```python
from build123d import *

# Parameters (mm, degrees)
PAD_DEPTH       = 36
SKETCH001_R     = 4.2
POCKET_DEPTH    = 28.001
SKETCH002_R     = 16.5
POCKET001_DEPTH = 10
POCKET002_DEPTH = 6.5
SKETCH004_R     = 11.25
POCKET003_DEPTH = 1.5
SKETCH005_R     = 2.7
POCKET004_DEPTH = 10
SKETCH006_R     = 4.75
POCKET005_DEPTH = 1
CHAMFER_SIZE    = 3
CHAMFER001_SIZE = 4
CHAMFER002_SIZE = 6
CHAMFER003_SIZE = 3
CHAMFER004_SIZE = 0.8
CHAMFER005_SIZE = 1
CHAMFER006_SIZE = 0.6
CHAMFER007_SIZE = 0.4


with BuildPart() as part:
    # Sketch (on XZ_Plane of Origin) → Pad (new body, symmetric)
    with BuildSketch(Plane.XZ):
        Polygon((0, 0), (0, 20), (-37, 20), (-37, -8), (20, -8), (20, 0), align=None)
    extrude(amount=PAD_DEPTH, both=True)

    # Sketch001 (on Face2 of Pad) → Pocket (cut, through all)
    with BuildSketch(Plane.XY.offset(20)):
        with Locations((-18.5, 0)):
            Circle(SKETCH001_R)
    extrude(amount=-POCKET_DEPTH, mode=Mode.SUBTRACT)

    # Sketch002 (on Face9 of Pocket) → Pocket001 (cut)
    with BuildSketch(Plane(origin=(0, 0, -8), x_dir=(1, 0, 0), z_dir=(0, 0, -1))):
        with Locations((-18.5, 0)):
            Circle(SKETCH002_R)
    extrude(amount=-POCKET001_DEPTH, mode=Mode.SUBTRACT)

    # Sketch003 (on Face10 of Pocket001) → Pocket002 (cut)
    with BuildSketch(Plane(origin=(0, 0, 2), x_dir=(1, 0, 0), z_dir=(0, 0, -1))):
        Polygon((-10.994447, 0), (-14.747223, 6.5), (-22.252777, 6.5), (-26.005553, 0), (-22.252777, -6.5), (-14.747223, -6.5), align=None)
    extrude(amount=-POCKET002_DEPTH, mode=Mode.SUBTRACT)

    # Sketch004 (on Face3 of Pocket002) → Pocket003 (cut)
    with BuildSketch(Plane.XY.offset(20)):
        with Locations((-18.5, 0)):
            Circle(SKETCH004_R)
    extrude(amount=-POCKET003_DEPTH, mode=Mode.SUBTRACT)

    # Sketch005 (on Face2 of Pocket003) → Pocket004 (cut)
    with BuildSketch(Plane.XY):
        with Locations((10, -26)):
            Circle(SKETCH005_R)
        with Locations((10, 26)):
            Circle(SKETCH005_R)
    extrude(amount=-POCKET004_DEPTH, mode=Mode.SUBTRACT)

    # Sketch006 (on Face11 of Pocket004) → Pocket005 (cut)
    with BuildSketch(Plane(origin=(0, 0, -8), x_dir=(1, 0, 0), z_dir=(0, 0, -1))):
        with Locations((10, 26)):
            Circle(SKETCH006_R)
        with Locations((10, -26)):
            Circle(SKETCH006_R)
    extrude(amount=-POCKET005_DEPTH, mode=Mode.SUBTRACT)

    # Chamfer
    chamfer_edges = [part.edges().sort_by_distance(p)[0] for p in [
        (0, -36, 10),
        (0, 36, 10),
    ]]
    chamfer(chamfer_edges, length=CHAMFER_SIZE)

    # Chamfer001
    chamfer001_edges = [part.edges().sort_by_distance(p)[0] for p in [
        (20, -36, -4),
        (20, 36, -4),
    ]]
    chamfer(chamfer001_edges, length=CHAMFER001_SIZE)

    # Chamfer002
    chamfer002_edges = [part.edges().sort_by_distance(p)[0] for p in [
        (-37, -36, 6),
        (-37, 36, 6),
    ]]
    chamfer(chamfer002_edges, length=CHAMFER002_SIZE)

    # Chamfer003
    chamfer003_edges = [part.edges().sort_by_distance(p)[0] for p in [
        (-35, 0, 2),
    ]]
    chamfer(chamfer003_edges, length=CHAMFER003_SIZE)

    # Chamfer004
    chamfer004_edges = [part.edges().sort_by_distance(p)[0] for p in [
        (-35, 0, -8),
    ]]
    chamfer(chamfer004_edges, length=CHAMFER004_SIZE)

    # Chamfer005
    chamfer005_edges = [part.edges().sort_by_distance(p)[0] for p in [
        (-22.7, 0, 18.5),
        (-22.7, 0, 8.5),
    ]]
    chamfer(chamfer005_edges, length=CHAMFER005_SIZE)

    # Chamfer006
    chamfer006_edges = [part.edges().sort_by_distance(p)[0] for p in [
        (7.3, 26, -7),
        (7.3, -26, -7),
        (7.3, -26, 0),
        (7.3, 26, 0),
    ]]
    chamfer(chamfer006_edges, length=CHAMFER006_SIZE)

    # Chamfer007
    chamfer007_edges = [part.edges().sort_by_distance(p)[0] for p in [
        (-17, 36, 20),
        (-34, 33, 20),
        (-1.5, 34.5, 20),
        (-37, 0, 20),
        (0, 0, 20),
        (-34, -33, 20),
        (-1.5, -34.5, 20),
        (-17, -36, 20),
        (-29.75, 0, 20),
        (-35.8, 0, -8),
        (-7.5, 36, -8),
        (-34, 33, -8),
        (18, 34, -8),
        (-37, 0, -8),
        (20, 0, -8),
        (-34, -33, -8),
        (18, -34, -8),
        (-7.5, -36, -8),
        (5.25, -26, -8),
        (5.25, 26, -8),
    ]]
    chamfer(chamfer007_edges, length=CHAMFER007_SIZE)


solid = part.part
```
Part model, mm, in its own coordinate system. A direction names the side the tool comes from. Round coordinates to 2 decimals unless told otherwise and drop trailing zeros. Order: outer loops, then holes, each group sorted by start corner. A loop starts at its lowest first (then second) coordinate and runs counter-clockwise, first axis right, second up. Notation, with made-up numbers: M 20.5,35 L 39.5,35 A30 ccw 39.5,58 Z; hole C 28.5,36 d4. An arc over 180 degrees is marked long. Put each result on its own line as item: value. Start each with the question number.
1. Slice it at C-C on z = 14. List the corners of the cut face in (x, y).
2. Slice it at B-B on x = 10. State how many separate pieces and enclosed holes the cut face has, then the cut area to 3 significant figures.
3. Drill centre lines: probe 1 along Y at (x, z) = (10, -3.6); probe 2 along Y at (x, z) = (10, -7.2); probe 3 along Y at (x, z) = (-18.5, 18.7). Where is each one in solid material? Low to high. Write a range as [from, to].
4. Drop flat-ended pins along their axis: pin 1 (7 mm diameter, centred on x = 8.5, y = -1, fed in from +Z); pin 2 (6.5 mm diameter, centred on x = -18.5, y = 0, fed in from +Z); pin 3 (6.5 mm diameter, centred on x = -17, y = -3, fed in from -Z); pin 4 (7 mm diameter, centred on x = 10, y = 26, fed in from -Z). Give the stop position or say it passes through.
5. Slice it at A-A on y = -26. List the corners of the cut face in (x, z).
6. Tool access for faces 1 (the face through (-2, 35, 10)), 2 (the face through (-14, 3, 8.5)), 3 (the face through (-2.6, -8.4, -8)), 4 (the face through (-16, -5, 18.5)), 5 (the face through (-33.82, 32.9, -7.8)): list every direction of +Z, -Z, +X, -X, +Y, -Y with a clear straight run to the whole face (end or side of a thin tool).
7. Two-plate mould, pull along Y, no slides. Class faces 6 (the face through (-37, 0, 6)), 7 (the face through (-33.82, -32.9, -7.8)), 8 (the face through (-27.428, -6.845, 19.058)): +Y half, -Y half, draft (parallel to the pull), parting line (faces both ways), or undercut.
Findings:
1. outline: M -37,-30 L -31,-36 L -3,-36 L 0,-33 L 0,33 L -3,36 L -31,36 L -37,30 Z; hole C -18.5,0 d8.4
2. separate pieces: 3
2. enclosed holes: 0
2. area: 479 mm2
3. probe 1: [-36, -28.7], [-23.3, 23.3], [28.7, 36]
3. probe 2: [-36, -30.75], [-21.25, 21.25], [30.75, 36]
3. probe 3: [-36, -11.25], [11.25, 36]
4. pin 1: z = 0
4. pin 2: through
4. pin 3: z = 8.5
4. pin 4: z = -7
5. outline: M -37,-7.6 L -36.6,-8 L 4.85,-8 L 5.25,-7.6 L 5.25,-7 L 6.7,-7 L 7.3,-6.4 L 7.3,-0.6 L 6.7,0 L 0,0 L 0,19.6 L -0.4,20 L -36.6,20 L -37,19.6 Z; M 12.7,-6.4 L 13.3,-7 L 14.75,-7 L 14.75,-7.6 L 15.15,-8 L 19.6,-8 L 20,-7.6 L 20,0 L 13.3,0 L 12.7,-0.6 Z
6. face 1: +Z, +X, +Y
6. face 2: -Z
6. face 3: -Z, +X, -X, +Y, -Y
6. face 4: +Z
6. face 5: -Z, -X, +Y
7. face 6: draft
7. face 7: -Y half
7. face 8: undercut
